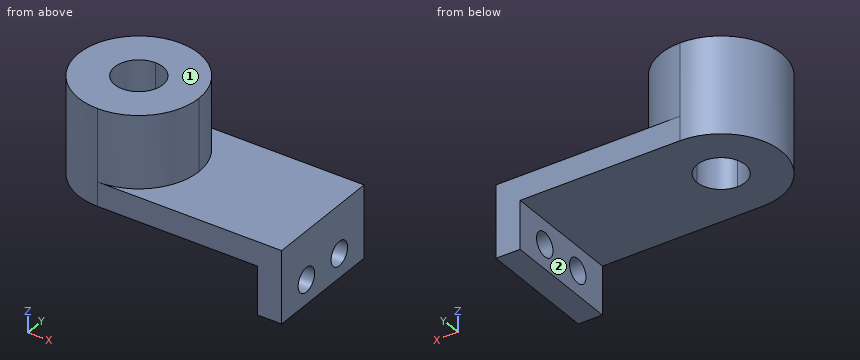
from build123d import *

# Parameters (mm, degrees)
F1_DEPTH = 12.7
F2_DEPTH = 50.8
F3_R     = 6.35
F4_DEPTH = 12.7


with BuildPart() as f1:
    # F0 (on Top) → F1 (new body)
    with BuildSketch(Plane.XY):
        with BuildLine():
            Line((-48.517924, -31.75), (48.517924, -31.75))
            Line((48.517924, -31.75), (48.517924, 31.75))
            Line((48.517924, 31.75), (-48.517924, 31.75))
            ThreePointArc((-48.517924, 31.75), (-26.067284, 22.45064), (-16.767924, 0))
            ThreePointArc((-16.767924, 0), (-26.067284, -22.45064), (-48.517924, -31.75))
        make_face()
        with BuildLine():
            ThreePointArc((-48.517924, 31.75), (-80.267924, 0), (-48.517924, -31.75))
            Line((-48.517924, -31.75), (-48.517924, -12.7))
            ThreePointArc((-48.517924, -12.7), (-61.217924, 0), (-48.517924, 12.7))
            Line((-48.517924, 12.7), (-48.517924, 31.75))
        make_face()
    extrude(amount=F1_DEPTH)

    # F0 (on Top) → F2 (join)
    with BuildSketch(Plane.XY):
        with BuildLine():
            Line((-48.517924, -12.7), (-48.517924, -31.75))
            ThreePointArc((-48.517924, -31.75), (-26.067284, -22.45064), (-16.767924, 0))
            ThreePointArc((-16.767924, 0), (-26.067284, 22.45064), (-48.517924, 31.75))
            Line((-48.517924, 31.75), (-48.517924, 12.7))
            ThreePointArc((-48.517924, 12.7), (-39.537668, 8.980256), (-35.817924, 0))
            ThreePointArc((-35.817924, 0), (-39.537668, -8.980256), (-48.517924, -12.7))
        make_face()
        with BuildLine():
            ThreePointArc((-48.517924, 31.75), (-80.267924, 0), (-48.517924, -31.75))
            Line((-48.517924, -31.75), (-48.517924, -12.7))
            ThreePointArc((-48.517924, -12.7), (-61.217924, 0), (-48.517924, 12.7))
            Line((-48.517924, 12.7), (-48.517924, 31.75))
        make_face()
    extrude(amount=F2_DEPTH)

    # F3 (on face) → F4 (join)
    with BuildSketch(Plane.YZ.offset(48.517924)):
        Polygon((31.75, 12.7), (-31.75, 12.7), (-31.75, -25.4), (0, -25.4), (31.75, -25.4), align=None)
        with Locations((-12.7, -12.7)):
            Circle(F3_R, mode=Mode.SUBTRACT)
        with Locations((12.7, -12.7)):
            Circle(F3_R, mode=Mode.SUBTRACT)
    extrude(amount=-F4_DEPTH)


solid = f1.part
Read the model definition and answer for the solid it produces. Units are mm, in the model's axes. Face numbers are marked on the shaded views. A direction names the side the tool comes from. Coordinates: 2 decimals unless noted, no trailing zeros. Order: outer loops, then holes, each group sorted by start corner. A loop starts at its lowest first (then second) coordinate and runs counter-clockwise, first axis right, second up. Notation, with made-up numbers: M 70.25,-27.5 L 103.25,-27.5 A29 cw 103.25,3.5 Z; hole C 3.5,60.25 d2. An arc over 180 degrees is marked long. Put each result on its own line as item: value. Start each with the question number.
Item 1: Section C-C, the plane z = -12.7 is taken. Determine the outline of the cut face in (x, y), plus the area to 3 significant figures.
Item 2: Given pin 1 Ø10 at (y, z) = (-0.5, 30.5) entering from -X; pin 2 Ø2 at (y, z) = (-25, -10) entering from -X; pin 3 Ø7.5 at (y, z) = (-12.7, -12.7) entering from +X; pin 4 Ø8 at (y, z) = (1, 27) entering from +X, each flat-ended and moving along its own axis, determine where each tip first touches the part or whether it passes through.
Item 3: Section B-B, the plane y = -10 is taken. Determine the outline of the cut face in (x, z), plus the area to 3 significant figures.
Item 4: Section A-A, the plane z = 10 is taken. Determine the outline of the cut face in (x, y), plus the area to 3 significant figures.
Item 5: Section D-D, the plane y = 1.5 is taken. Determine the outline of the cut face in (x, z), plus the area to 3 significant figures.
Item 6: For the marked faces 1 and 2, determine the directions among +Z, -Z, +X, -X, +Y, -Y from which every point of the face is accessible in a straight line to the end or side of a thin tool.
Item 7: Consider probe 1 along Z at (x, y) = (40.75, -12.7); probe 2 along Y at (x, z) = (38, -12); probe 3 along Z at (x, y) = (-44.5, 20). Determine where each line is inside the solid, lowest interval first. Write a range as [from, to].
Computed:
1. outline: M 35.82,-31.75 L 48.52,-31.75 L 48.52,-19.05 L 35.82,-19.05 Z; M 35.82,-6.35 L 48.52,-6.35 L 48.52,6.35 L 35.82,6.35 Z; M 35.82,19.05 L 48.52,19.05 L 48.52,31.75 L 35.82,31.75 Z
1. area: 484 mm2
2. pin 1: stops at x = -80.27
2. pin 2: stops at x = 35.82
2. pin 3: passes through
2. pin 4: stops at x = -16.77
3. outline: M -78.65,0 L -56.35,0 L -56.35,50.8 L -78.65,50.8 Z; M -40.69,0 L 35.82,0 L 35.82,-6.95 L 48.52,-6.95 L 48.52,12.7 L -18.38,12.7 L -18.38,50.8 L -40.69,50.8 Z; M 35.82,-25.4 L 48.52,-25.4 L 48.52,-18.45 L 35.82,-18.45 Z
3. area: 3,290 mm2
4. outline: M -48.52,-31.75 L 48.52,-31.75 L 48.52,31.75 L -48.52,31.75 A31.75 ccw Z; hole C -48.52,0 d25.4
4. area: 7,240 mm2
5. outline: M -80.23,0 L -61.13,0 L -61.13,50.8 L -80.23,50.8 Z; M -35.91,0 L 35.82,0 L 35.82,-25.4 L 48.52,-25.4 L 48.52,12.7 L -16.8,12.7 L -16.8,50.8 L -35.91,50.8 Z
5. area: 3,090 mm2
6. face 1: +Z, +X, -X, +Y, -Y
6. face 2: -Z, -X, +Y, -Y
7. probe 1: z = [-25.4, -19.05], [-6.35, 12.7]
7. probe 2: y = [-31.75, -19.01], [-6.39, 6.39], [19.01, 31.75]
7. probe 3: z = [0, 50.8]
